from build123d import *

# Parameters (mm, degrees)
SKETCH_1_W      = 200
SKETCH_1_H      = 385
SKETCH_1_R      = 7.90569415
SKETCH_1_R_2    = 1.65
SKETCH_1_R_3    = 1.75
EXTRUDE_1_DEPTH = 5
FILLET_1_R      = 5


with BuildPart() as part:
    # 草图1 → 凸台-拉伸1 (new body)
    with BuildSketch(Plane.XY):
        Rectangle(SKETCH_1_W, SKETCH_1_H)
        with Locations((-80, 180)):
            Circle(SKETCH_1_R, mode=Mode.SUBTRACT)
        with Locations((-80, 0)):
            Circle(SKETCH_1_R, mode=Mode.SUBTRACT)
        with Locations((-80, -180)):
            Circle(SKETCH_1_R, mode=Mode.SUBTRACT)
        with Locations((80, -180)):
            Circle(SKETCH_1_R, mode=Mode.SUBTRACT)
        with Locations((80, 0)):
            Circle(SKETCH_1_R, mode=Mode.SUBTRACT)
        with Locations((80, 180)):
            Circle(SKETCH_1_R, mode=Mode.SUBTRACT)
        with Locations((-30, 174.165738454)):
            Circle(SKETCH_1_R_2, mode=Mode.SUBTRACT)
        with Locations((-30, 151.165738454)):
            Circle(SKETCH_1_R_2, mode=Mode.SUBTRACT)
        with Locations((-30, 128.165738454)):
            Circle(SKETCH_1_R_2, mode=Mode.SUBTRACT)
        with Locations((-62, 128.165738454)):
            Circle(SKETCH_1_R_2, mode=Mode.SUBTRACT)
        with Locations((-62, 151.165738454)):
            Circle(SKETCH_1_R_2, mode=Mode.SUBTRACT)
        with Locations((-62, 174.165738454)):
            Circle(SKETCH_1_R_2, mode=Mode.SUBTRACT)
        with Locations((-30, -5.702436416)):
            Circle(SKETCH_1_R_2, mode=Mode.SUBTRACT)
        with Locations((-30, -28.702436416)):
            Circle(SKETCH_1_R_2, mode=Mode.SUBTRACT)
        with Locations((-30, -51.702436416)):
            Circle(SKETCH_1_R_2, mode=Mode.SUBTRACT)
        with Locations((-62, -51.702436416)):
            Circle(SKETCH_1_R_2, mode=Mode.SUBTRACT)
        with Locations((-62, -28.702436416)):
            Circle(SKETCH_1_R_2, mode=Mode.SUBTRACT)
        with Locations((-62, -5.702436416)):
            Circle(SKETCH_1_R_2, mode=Mode.SUBTRACT)
        with Locations((30, -128.126766598)):
            Circle(SKETCH_1_R_2, mode=Mode.SUBTRACT)
        with Locations((30, -151.126766598)):
            Circle(SKETCH_1_R_2, mode=Mode.SUBTRACT)
        with Locations((30, -174.126766598)):
            Circle(SKETCH_1_R_2, mode=Mode.SUBTRACT)
        with Locations((62, -174.126766598)):
            Circle(SKETCH_1_R_2, mode=Mode.SUBTRACT)
        with Locations((62, -151.126766598)):
            Circle(SKETCH_1_R_2, mode=Mode.SUBTRACT)
        with Locations((62, -128.126766598)):
            Circle(SKETCH_1_R_2, mode=Mode.SUBTRACT)
        with Locations((-30, -148.12043677)):
            Circle(SKETCH_1_R_2, mode=Mode.SUBTRACT)
        with Locations((-30, -171.12043677)):
            Circle(SKETCH_1_R_2, mode=Mode.SUBTRACT)
        with Locations((-62, -171.12043677)):
            Circle(SKETCH_1_R_2, mode=Mode.SUBTRACT)
        with Locations((-62, -148.12043677)):
            Circle(SKETCH_1_R_2, mode=Mode.SUBTRACT)
        with Locations((30, 13.14999216)):
            Circle(SKETCH_1_R_2, mode=Mode.SUBTRACT)
        with Locations((30, -9.85000784)):
            Circle(SKETCH_1_R_2, mode=Mode.SUBTRACT)
        with Locations((30, -32.85000784)):
            Circle(SKETCH_1_R_2, mode=Mode.SUBTRACT)
        with Locations((62, -32.85000784)):
            Circle(SKETCH_1_R_2, mode=Mode.SUBTRACT)
        with Locations((62, -9.85000784)):
            Circle(SKETCH_1_R_2, mode=Mode.SUBTRACT)
        with Locations((62, 13.14999216)):
            Circle(SKETCH_1_R_2, mode=Mode.SUBTRACT)
        with Locations((30, 171.131672491)):
            Circle(SKETCH_1_R_2, mode=Mode.SUBTRACT)
        with Locations((30, 148.131672491)):
            Circle(SKETCH_1_R_2, mode=Mode.SUBTRACT)
        with Locations((62, 148.131672491)):
            Circle(SKETCH_1_R_2, mode=Mode.SUBTRACT)
        with Locations((62, 171.131672491)):
            Circle(SKETCH_1_R_2, mode=Mode.SUBTRACT)
        with Locations((89.5, -170.5)):
            Circle(SKETCH_1_R_3, mode=Mode.SUBTRACT)
        with Locations((89.5, -189.5)):
            Circle(SKETCH_1_R_3, mode=Mode.SUBTRACT)
        with Locations((70.5, -189.5)):
            Circle(SKETCH_1_R_3, mode=Mode.SUBTRACT)
        with Locations((70.5, -170.5)):
            Circle(SKETCH_1_R_3, mode=Mode.SUBTRACT)
        with Locations((-70.5, -170.5)):
            Circle(SKETCH_1_R_3, mode=Mode.SUBTRACT)
        with Locations((-70.5, -189.5)):
            Circle(SKETCH_1_R_3, mode=Mode.SUBTRACT)
        with Locations((-89.5, -189.5)):
            Circle(SKETCH_1_R_3, mode=Mode.SUBTRACT)
        with Locations((-89.5, -170.5)):
            Circle(SKETCH_1_R_3, mode=Mode.SUBTRACT)
        with Locations((89.5, -9.5)):
            Circle(SKETCH_1_R_3, mode=Mode.SUBTRACT)
        with Locations((70.5, -9.5)):
            Circle(SKETCH_1_R_3, mode=Mode.SUBTRACT)
        with Locations((89.5, 9.5)):
            Circle(SKETCH_1_R_3, mode=Mode.SUBTRACT)
        with Locations((70.5, 9.5)):
            Circle(SKETCH_1_R_3, mode=Mode.SUBTRACT)
        with Locations((89.5, 170.5)):
            Circle(SKETCH_1_R_3, mode=Mode.SUBTRACT)
        with Locations((70.5, 170.5)):
            Circle(SKETCH_1_R_3, mode=Mode.SUBTRACT)
        with Locations((89.5, 189.5)):
            Circle(SKETCH_1_R_3, mode=Mode.SUBTRACT)
        with Locations((70.5, 189.5)):
            Circle(SKETCH_1_R_3, mode=Mode.SUBTRACT)
        with Locations((-70.5, 170.5)):
            Circle(SKETCH_1_R_3, mode=Mode.SUBTRACT)
        with Locations((-89.5, 170.5)):
            Circle(SKETCH_1_R_3, mode=Mode.SUBTRACT)
        with Locations((-70.5, 189.5)):
            Circle(SKETCH_1_R_3, mode=Mode.SUBTRACT)
        with Locations((-89.5, 189.5)):
            Circle(SKETCH_1_R_3, mode=Mode.SUBTRACT)
        with Locations((-89.5, -9.5)):
            Circle(SKETCH_1_R_3, mode=Mode.SUBTRACT)
        with Locations((-70.5, -9.5)):
            Circle(SKETCH_1_R_3, mode=Mode.SUBTRACT)
        with Locations((-70.5, 9.5)):
            Circle(SKETCH_1_R_3, mode=Mode.SUBTRACT)
        with Locations((-89.5, 9.5)):
            Circle(SKETCH_1_R_3, mode=Mode.SUBTRACT)
    extrude(amount=EXTRUDE_1_DEPTH)

    # 圆角1
    fillet_1_edges = [part.edges().sort_by_distance(p)[0] for p in [
        (-100, 192.5, 2.5),
        (100, 192.5, 2.5),
        (100, -192.5, 2.5),
        (-100, -192.5, 2.5),
    ]]
    fillet(fillet_1_edges, radius=FILLET_1_R)


solid = part.part
Work out the finished part from the listing and answer in its coordinate system (mm). Round coordinates to 2 decimals unless told otherwise and drop trailing zeros. Write each loop counter-clockwise with the first axis right and the second up, starting at its lowest first coordinate (ties: lowest second). Pieces come first, ordered by that corner, then holes. Notation, with made-up numbers: (55.25, -28) -> (90.25, -28) arc R18 cw to (90.25, -8) -> close; hole circle Ø10 at (54.5, -25). An arc over 180 degrees is marked (long way). Answer as CSV lines item,"result". Start each with the question number.
(1) The part is cut by section C-C, the plane z = 2.9. Give the number of separate pieces and of enclosed holes in the cut face, then the cut area to 3 significant figures.
(2) This flat-tipped pin is pushed along its axis until it touches: pin 1 (5.5 mm diameter, centred on x = 30, y = -151.13, fed in from +Z). Where does it stop, or does it pass through?
(3) The part is cut by section B-B, the plane x = -79.5. Give the vertices of the cut face in (y, z).
(4) The mould has two halves that part along X. Classify faces 1 (the flat face through (-1, 3, 0)), 2 (the cylindrical face through (84.25, 186.666, 2.465)): +X half, -X half, draft (parallel to the pull), parting line (faces both ways), or undercut.
(5) Find the intervals of material crossed by probe 1 along X at (y, z) = (12, 0.45); probe 2 along X at (y, z) = (-189.5, 3.3); probe 3 along Y at (x, z) = (-79.5, 0.5), in increasing order.
(6) The part is cut by section A-A, the plane x = 80. Give the vertices of the cut face in (y, z), then the cut area to 3 significant figures.
Output values:
1,separate pieces,"1"
1,enclosed holes,"62"
1,area,"75,300 mm²"
2,pin 1,"stops at z = 5"
3,outline,"(-192.5, 0) -> (-187.89, 0) -> (-187.89, 5) -> (-192.5, 5) -> close; (-172.11, 0) -> (-7.89, 0) -> (-7.89, 5) -> (-172.11, 5) -> close; (7.89, 0) -> (172.11, 0) -> (172.11, 5) -> (7.89, 5) -> close; (187.89, 0) -> (192.5, 0) -> (192.5, 5) -> (187.89, 5) -> close"
4,face 1,"draft"
4,face 2,"undercut"
5,probe 1,"x = -100 to 28.82, 31.18 to 60.82, 63.18 to 100"
5,probe 2,"x = -99.58 to -91.25, -87.75 to -72.25, -68.75 to 68.75, 72.25 to 87.75, 91.25 to 99.58"
5,probe 3,"y = -192.5 to -187.89, -172.11 to -7.89, 7.89 to 172.11, 187.89 to 192.5"
6,outline,"(-192.5, 0) -> (-187.91, 0) -> (-187.91, 5) -> (-192.5, 5) -> close; (-172.09, 0) -> (-7.91, 0) -> (-7.91, 5) -> (-172.09, 5) -> close; (7.91, 0) -> (172.09, 0) -> (172.09, 5) -> (7.91, 5) -> close; (187.91, 0) -> (192.5, 0) -> (192.5, 5) -> (187.91, 5) -> close"
6,area,"1,690 mm²"
